The figure shows three views and two pictorial views of one solid part (mm, origin at its lowest corner). Answer the questions. A direction names the side the tool comes from. Coordinates: 2 decimals unless noted, no trailing zeros. Write each loop counter-clockwise with the first axis right and the second up, starting at its lowest first coordinate (ties: lowest second). Pieces come first, ordered by that corner, then holes.
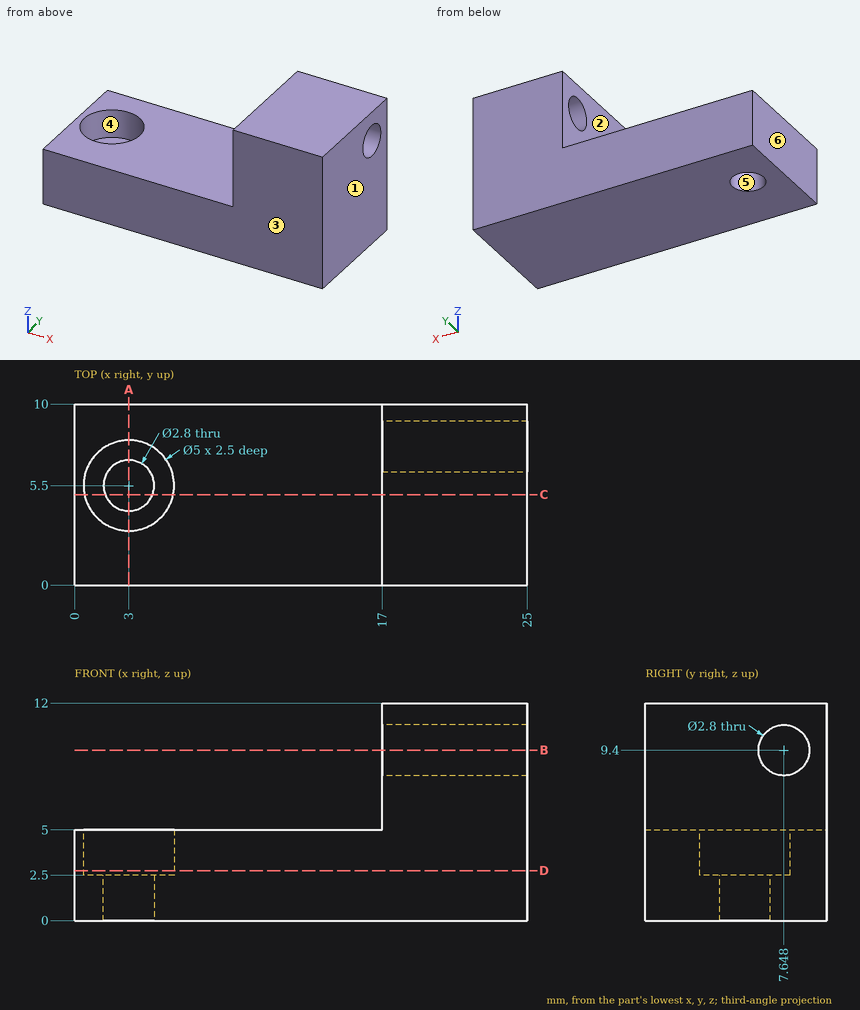
Q1. Given pin 1 (4.5 mm diameter, centred on x = 3, y = 5.5, fed in from +Z); pin 2 (2 mm diameter, centred on x = 5.5, y = 2.5, fed in from +Z); pin 3 (1.5 mm diameter, centred on y = 7, z = 4.5, fed in from -X); pin 4 (2 mm diameter, centred on y = 6.5, z = 8, fed in from -X), each flat-ended and moving along its own axis, determine where each tip first touches the part or whether it passes through.
Answers below:
pin 1: stops at z = 2.5
pin 2: stops at z = 5
pin 3: stops at x = 0
pin 4: stops at x = 17
Q2. The part is cut by section A-A, the plane x = 3. Write down the section's boundary in (y, z), then the cut area to 3 significant figures.
Answers below:
outline: (0, 0) - (4.1, 0) - (4.1, 2.5) - (3, 2.5) - (3, 5) - (0, 5) - close; (6.9, 0) - (10, 0) - (10, 5) - (8, 5) - (8, 2.5) - (6.9, 2.5) - close
area: 30.5 mm2
Q3. Which of the six approach directions +Z, -Z, +X, -X, +Y, -Y give full straight-line access (tool end or side, diameter ignored) to the marked faces 1 and 2?
Answers below:
face 1: +Z, -Z, +X, +Y, -Y
face 2: +Z, -X, +Y, -Y
Q4. The part is cut by section C-C, the plane y = 5. Write down the section's boundary in (x, z).
Answers below:
outline: (0, 0) - (1.69, 0) - (1.69, 2.5) - (0.55, 2.5) - (0.55, 5) - (0, 5) - close; (4.31, 0) - (25, 0) - (25, 12) - (17, 12) - (17, 5) - (5.45, 5) - (5.45, 2.5) - (4.31, 2.5) - close
Q5. The part is cut by section D-D, the plane z = 2.75. Write down the section's boundary in (x, y), then the cut area to 3 significant figures.
Answers below:
outline: (0, 0) - (25, 0) - (25, 10) - (0, 10) - close; hole circle Ø5 at (3, 5.5)
area: 230 mm2
Q6. The part is cut by section B-B, the plane z = 9.4. Write down the section's boundary in (x, y), then the cut area to 3 significant figures.
Answers below:
outline: (17, 0) - (25, 0) - (25, 6.25) - (17, 6.25) - close; (17, 9.05) - (25, 9.05) - (25, 10) - (17, 10) - close
area: 57.6 mm2
Q7. Find the intervals of material crossed by probe 1 along Y at (x, z) = (3, 3.35); probe 2 along Y at (x, z) = (3, 1.8); probe 3 along Z at (x, y) = (6.25, 4.25), in increasing order.
Answers below:
probe 1: y = 0 to 3, 8 to 10
probe 2: y = 0 to 4.1, 6.9 to 10
probe 3: z = 0 to 5
Q8. Determine the mould class of the marked faces 3, 4, 5 and 6 for opening direction X: released by +X, released by -X, zero draft, split by the parting line, or undercut.
Answers below:
face 3: zero draft
face 4: undercut
face 5: undercut
face 6: released by -X
